Build history of the part. All positions in model axes, mm. A direction names the side the tool comes from. Round coordinates to 2 decimals unless told otherwise and drop trailing zeros. Write each loop counter-clockwise with the first axis right and the second up, starting at its lowest first coordinate (ties: lowest second). Pieces come first, ordered by that corner, then holes.
from build123d import *

# Parameters (mm, degrees)
ROTATION1_ANGLE                      = 20
SCHNITT_LINEAR_AUSTRAGEN2_DEPTH      = 15.24
SCHNITT_LINEAR_AUSTRAGEN2_DEPTH_BACK = 2.54


with BuildPart() as part:
    # Skizze1 → Rotation1 (revolve, symmetric)
    with BuildSketch(Plane(origin=(0, 0, 0), x_dir=(0, 0, -1), z_dir=(1, 0, 0))) as rotation1_sk:
        Polygon((0, 161.09315), (68.208324134, 177.5), (90, 177.5), (90, 165), (70.634410551, 165), (2.974994021, 148.725184394), align=None)
    revolve(axis=Axis((0, 0, 0), (0, 0, -1)), revolution_arc=ROTATION1_ANGLE / 2)
    revolve(rotation1_sk.sketch, axis=Axis((0, 0, 0), (0, 0, 1)), revolution_arc=ROTATION1_ANGLE / 2)

    # Skizze4 → Schnitt-Linear austragen2 (cut, two sides)
    with BuildSketch(Plane(origin=(0, 169.424608185, -38.218632457), x_dir=(-1, 0, 0), z_dir=(0, -0.978056789, -0.208338468))) as schnitt_linear_austragen2_sk:
        with BuildLine():
            Line((12.109444482, 32.004), (-12.109444482, 32.004))
            ThreePointArc((-12.109444482, 32.004), (-12.895155782, 32.226245034), (-13.448039836, 32.827122995))
            ThreePointArc((-13.448039836, 32.827122995), (-17.173364468, 34.441533799), (-19.440102095, 31.073111855))
            Line((-19.440102095, 31.073111855), (-17.558493636, -29.330115121))
            ThreePointArc((-17.558493636, -29.330115121), (-16.083752787, -32.838011315), (-12.302447063, -32.411486631))
            ThreePointArc((-12.302447063, -32.411486631), (-11.827451319, -32.109587928), (-11.274626778, -32.004))
            Line((-11.274626778, -32.004), (11.274626778, -32.004))
            ThreePointArc((11.274626778, -32.004), (11.827451319, -32.109587928), (12.302447063, -32.411486631))
            ThreePointArc((12.302447063, -32.411486631), (16.083752787, -32.838011315), (17.558493636, -29.330115121))
            Line((17.558493636, -29.330115121), (19.440102095, 31.073111855))
            ThreePointArc((19.440102095, 31.073111855), (17.173364468, 34.441533799), (13.448039836, 32.827122995))
            ThreePointArc((13.448039836, 32.827122995), (12.895155782, 32.226245034), (12.109444482, 32.004))
        make_face()
    extrude(amount=SCHNITT_LINEAR_AUSTRAGEN2_DEPTH, mode=Mode.SUBTRACT)
    extrude(schnitt_linear_austragen2_sk.sketch, amount=-SCHNITT_LINEAR_AUSTRAGEN2_DEPTH_BACK, mode=Mode.SUBTRACT)


solid = part.part
1) Slice it at A-A (z = -42). Write the cut outline in (x, y) (3 decimals), plus the area to 3 significant figures.
Results:
outline: (-29.728, 168.595) - (-27.456, 155.71) arc R158.112 cw to (-18.507, 157.025) - (-18.592, 170.183) arc R171.196 ccw to start; (18.507, 157.025) arc R158.112 cw to (27.456, 155.71) - (29.728, 168.595) arc R171.196 ccw to (18.592, 170.183) - close
area: 266 mm2
2) Pin check, flat tips, straight feed: pin 1 Ø10 at (x, y) = (1.5, 156.5) entering from -Z; pin 2 Ø1.5 at (x, z) = (-24, -33.5) entering from +Y; pin 3 Ø1.5 at (x, y) = (-17, 173.5) entering from +Z; pin 4 Ø5 at (x, z) = (14, -17) entering from +Y. Stop position of each tip, or through.
Results:
pin 1: stops at z = -9.31
pin 2: stops at y = 167.65
pin 3: stops at z = -72.3
pin 4: passes through
3) Slice it at B-B (z = -53.5). Write the cut outline in (x, y), plus the area to 3 significant figures.
Results:
outline: (-30.21, 171.32) - (-27.94, 158.43) arc R160.88 cw to (-18.88, 159.77) - (-18.96, 172.93) arc R173.96 ccw to start; (18.88, 159.77) arc R160.88 cw to (27.94, 158.43) - (30.21, 171.32) arc R173.96 ccw to (18.96, 172.93) - close
area: 269 mm2
4) Wall check: L1, parallel to X at y = 160, z = -49; L2, parallel to X at y = 169, z = -71; L3, parallel to Z at x = -2.5, y = 157. Give the ranges that are in metal, low to high.
Results:
L1: x = -28.21 to -18.74, 18.74 to 28.21
L2: x = -29.8 to -19.4, 19.4 to 29.8
L3: z = -8.14 to -0.98
5) Which spindle directions (+Z, -Z, +X, -X, +Y, -Y) get a long thin tool onto all of the face, cutting with end or side? Do faces 1 (the flat face through (0.158, 156.423, -8.266)), 2 (the cylindrical face through (0, 165, -80)), 3 (the flat face through (-0.17, 170.937, -70.619)), 4 (the cylindrical face through (0.4, 177.5, -79.3)). Say none if no direction does.
Results:
face 1: -Z, +Y
face 2: -Z, -Y
face 3: +Z, -Y
face 4: +Z, -Z, +Y
